Here's how the part is built. I have some questions about the finished solid (model axes, mm). Coordinates: 2 decimals unless noted, no trailing zeros. Write each loop counter-clockwise with the first axis right and the second up, starting at its lowest first coordinate (ties: lowest second). Pieces come first, ordered by that corner, then holes.
Item 1: If we section it at C-C (x = 87.5): Please give me the cut outline in (y, z), then the cut area to 3 significant figures.
Item 2: If we section it at D-D (y = -201): Please give me the cut outline in (x, z), then the cut area to 3 significant figures.
Item 3: If we section it at B-B (z = -5.75): Count the separate pieces of the cut face and the enclosed holes in it, then the cut area to 3 significant figures.
Item 4: If we section it at A-A (y = -51): Please give me the cut outline in (x, z), then the cut area to 3 significant figures.
Item 5: If I drill on line 1 (Y direction, x = -85, z = -8); line 2 (X direction, y = 40, z = -3.5); line 3 (Y direction, x = 7.5, z = -13.5), over which ranges is the centre line in solid material (lowest first)?
Item 6: I'm going to push flat-ended pins straight in: pin 1 Ø3 at (x, z) = (-165, -14) entering from -Y; pin 2 Ø5.5 at (x, z) = (-5.5, -7) entering from +Y; pin 3 Ø5 at (y, z) = (56, -4) entering from -X. Where does each tip first touch, or does it pass through?
from build123d import *

# Parameters (mm, degrees)
F2_DEPTH  = 31.75
F4_DEPTH  = 11.43
F6_DEPTH  = 8.89
F8_DEPTH  = 8.89
F10_DEPTH = 8.89
F12_DEPTH = 8.89
F13_R     = 304.8
F14_DEPTH = 20.32
F16_DEPTH = 10.16
F18_DEPTH = 10.16
F20_DEPTH = 10.16
F22_DEPTH = 10.16
F24_DEPTH = 10.16
F26_DEPTH = 10.16
F27_R     = 304.8
F28_DEPTH = 38.1


with BuildPart() as f2:
    # F1 (on Top) → F2 (new body)
    with BuildSketch(Plane.XY):
        with BuildLine():
            ThreePointArc((-0.430908, 226.982415), (-79.711548, 181.706479), (-169.227302, 163.75488))
            Line((-169.227302, 163.75488), (-169.227302, -60.819823))
            ThreePointArc((-169.227302, -60.819823), (-113.369381, -185.600772), (2.933838, -257.461429))
            ThreePointArc((2.933838, -257.461429), (118.158195, -186.267639), (169.227302, -60.819823))
            Line((169.227302, -60.819823), (169.227302, 166.105464))
            ThreePointArc((169.227302, 166.105464), (79.251051, 182.199338), (-0.430908, 226.982415))
        make_face()
    extrude(amount=F2_DEPTH)

    # F3 (on face) → F4 (cut)
    with BuildSketch(Plane.XY.offset(31.75)):
        with BuildLine():
            ThreePointArc((-0.374756, 195.493162), (-69.015087, 155.212384), (-147.227302, 140.485346))
            Line((-147.227302, 140.485346), (-147.227302, -60.819823))
            ThreePointArc((-147.227302, -60.819823), (-96.87236, -165.644499), (2.548859, -225.97073))
            ThreePointArc((2.548859, -225.97073), (100.066402, -165.452439), (147.227302, -60.819823))
            Line((147.227302, -60.819823), (147.227302, 142.530277))
            ThreePointArc((147.227302, 142.530277), (68.839046, 156.227594), (-0.374756, 195.493162))
        make_face()
        with BuildLine():
            Line((-132.618561, -60.819823), (-135.227293, 127.792969))
            ThreePointArc((-135.227293, 127.792969), (-63.429471, 141.425292), (-0.343994, 178.316891))
            ThreePointArc((-0.343994, 178.316891), (63.444172, 142.853346), (135.227293, 129.670903))
            Line((135.227293, 129.670903), (135.227293, -60.819823))
            ThreePointArc((135.227293, -60.819823), (90.906741, -154.674215), (2.340942, -208.794981))
            ThreePointArc((2.340942, -208.794981), (-88.121088, -155.768197), (-132.618561, -60.819823))
        make_face(mode=Mode.SUBTRACT)
    extrude(amount=-F4_DEPTH, mode=Mode.SUBTRACT)

    # F5 (on face) → F6 (cut)
    with BuildSketch(Plane.XY.offset(31.75)):
        with BuildLine():
            Line((-92.367917, 113.127932), (-45.701414, 36.461424))
            Line((-45.701414, 36.461424), (53.798582, 36.461424))
            Line((53.798582, 36.461424), (100.798585, 113.127932))
            ThreePointArc((100.798585, 113.127932), (80.575922, 103.064845), (63.631594, 88.127926))
            ThreePointArc((63.631594, 88.127926), (53.573391, 92.641146), (42.631593, 91.29443))
            ThreePointArc((42.631593, 91.29443), (54.451081, 69.882064), (36.776334, 52.976649))
            ThreePointArc((36.776334, 52.976649), (17.177594, 68.050279), (25.131593, 91.460936))
            ThreePointArc((25.131593, 91.460936), (17.890886, 96.996315), (8.798584, 97.627439))
            ThreePointArc((8.798584, 97.627439), (11.159805, 118.634697), (4.798584, 138.794437))
            ThreePointArc((4.798584, 138.794437), (-2.905563, 118.768028), (-0.36792, 97.461425))
            ThreePointArc((-0.36792, 97.461425), (-9.949798, 97.0895), (-17.034912, 90.627931))
            ThreePointArc((-17.034912, 90.627931), (-9.141713, 67.277349), (-29.217625, 52.976649))
            ThreePointArc((-29.217625, 52.976649), (-46.671559, 70.152552), (-34.034912, 91.127932))
            ThreePointArc((-34.034912, 91.127932), (-45.151665, 92.60432), (-55.201415, 87.627932))
            ThreePointArc((-55.201415, 87.627932), (-71.812791, 103.251959), (-92.367917, 113.127932))
        make_face()
    extrude(amount=-F6_DEPTH, mode=Mode.SUBTRACT)

    # F7 (on face) → F8 (cut)
    with BuildSketch(Plane.XY.offset(31.75)):
        Polygon((1.882065, 29.461427), (67.46655, -21.70459), (47.798585, 29.461427), align=None)
    extrude(amount=-F8_DEPTH, mode=Mode.SUBTRACT)

    # F9 (on face) → F10 (cut)
    with BuildSketch(Plane.XY.offset(31.75)):
        Polygon((1.048598, 29.461427), (-44.867922, 29.461427), (-64.53491, -21.70459), align=None)
    extrude(amount=-F10_DEPTH, mode=Mode.SUBTRACT)

    # F11 (on face) → F12 (cut)
    with BuildSketch(Plane.XY.offset(31.75)):
        with BuildLine():
            Line((1.246826, -2.287598), (-12.11792, -13.121582))
            Line((-12.11792, -13.121582), (-17.534912, -87.538578))
            Line((-17.534912, -87.538578), (-27.712647, -87.456539))
            ThreePointArc((-27.712647, -87.456539), (-43.153284, -84.398915), (-38.845949, -99.538572))
            Line((-38.845949, -99.538572), (-9.99292, -99.538572))
            Line((-9.99292, -99.538572), (-10.230225, -136.209473))
            Line((-10.230225, -136.209473), (-16.215088, -143.374518))
            Line((-16.215088, -143.374518), (-10.201416, -149.538577))
            Line((-10.201416, -149.538577), (-3.201416, -149.538577))
            ThreePointArc((-3.201416, -149.538577), (-5.538014, -164.476042), (1.798584, -177.695796))
            ThreePointArc((1.798584, -177.695796), (7.646569, -164.237988), (6.611084, -149.601072))
            Line((6.611084, -149.601072), (11.986084, -149.476081))
            Line((11.986084, -149.476081), (19.017333, -143.569827))
            Line((19.017333, -143.569827), (12.298584, -136.203617))
            Line((12.298584, -136.203617), (12.131592, -99.538572))
            Line((12.131592, -99.538572), (41.065186, -99.538572))
            ThreePointArc((41.065186, -99.538572), (45.517328, -84.304241), (29.96753, -87.48389))
            Line((29.96753, -87.48389), (19.965576, -87.538578))
            Line((19.965576, -87.538578), (14.132569, -12.705078))
            Line((14.132569, -12.705078), (1.246826, -2.287598))
        make_face()
    extrude(amount=-F12_DEPTH, mode=Mode.SUBTRACT)

    # F13 (on face) → F14 (join)
    with BuildSketch(Plane.XY):
        with Locations((1.490798, -15.673031)):
            Circle(F13_R)
    extrude(amount=-F14_DEPTH)

    # F15 (on face) → F16 (cut)
    with BuildSketch(Plane.XY):
        with BuildLine():
            Line((-189.547302, 184.049582), (-189.547302, -62.041552))
            ThreePointArc((-189.547302, -62.041552), (-127.393416, -200.419297), (2.747771, -278.360156))
            ThreePointArc((2.747771, -278.360156), (132.255423, -201.050673), (189.547302, -61.527812))
            Line((189.547302, -61.527812), (189.547302, 187.032623))
            ThreePointArc((189.547302, 187.032623), (87.662532, 200.775305), (-0.410603, 253.808226))
            ThreePointArc((-0.410603, 253.808226), (-88.09635, 200.268094), (-189.547302, 184.049582))
        make_face()
        with BuildLine():
            Line((-169.227302, -60.819823), (-169.227302, 163.75488))
            ThreePointArc((-169.227302, 163.75488), (-79.711548, 181.706479), (-0.430908, 226.982415))
            ThreePointArc((-0.430908, 226.982415), (79.251051, 182.199338), (169.227302, 166.105464))
            Line((169.227302, 166.105464), (169.227302, -60.819823))
            ThreePointArc((169.227302, -60.819823), (118.158195, -186.267639), (2.933838, -257.461429))
            ThreePointArc((2.933838, -257.461429), (-113.369381, -185.600772), (-169.227302, -60.819823))
        make_face(mode=Mode.SUBTRACT)
    extrude(amount=-F16_DEPTH, mode=Mode.SUBTRACT)

    # F17 (on face) → F18 (cut)
    with BuildSketch(Plane.XY):
        with BuildLine():
            ThreePointArc((-0.374756, 195.493162), (-69.015087, 155.212384), (-147.227302, 140.485346))
            Line((-147.227302, 140.485346), (-147.227302, -60.819823))
            ThreePointArc((-147.227302, -60.819823), (-96.87236, -165.644499), (2.548859, -225.97073))
            ThreePointArc((2.548859, -225.97073), (100.066402, -165.452439), (147.227302, -60.819823))
            Line((147.227302, -60.819823), (147.227302, 142.530277))
            ThreePointArc((147.227302, 142.530277), (68.839046, 156.227594), (-0.374756, 195.493162))
        make_face()
        with BuildLine():
            Line((-132.618561, -60.819823), (-135.227293, 127.792969))
            ThreePointArc((-135.227293, 127.792969), (-63.429471, 141.425292), (-0.343994, 178.316891))
            ThreePointArc((-0.343994, 178.316891), (63.444172, 142.853346), (135.227293, 129.670903))
            Line((135.227293, 129.670903), (135.227293, -60.819823))
            ThreePointArc((135.227293, -60.819823), (90.906741, -154.674215), (2.340942, -208.794981))
            ThreePointArc((2.340942, -208.794981), (-88.121088, -155.768197), (-132.618561, -60.819823))
        make_face(mode=Mode.SUBTRACT)
    extrude(amount=-F18_DEPTH, mode=Mode.SUBTRACT)

    # F19 (on face) → F20 (cut)
    with BuildSketch(Plane.XY):
        with BuildLine():
            Line((19.965576, -87.538578), (14.132569, -12.705078))
            Line((14.132569, -12.705078), (1.246826, -2.287598))
            Line((1.246826, -2.287598), (-12.11792, -13.121582))
            Line((-12.11792, -13.121582), (-17.534912, -87.538578))
            Line((-17.534912, -87.538578), (-27.712647, -87.456539))
            ThreePointArc((-27.712647, -87.456539), (-43.153284, -84.398915), (-38.845949, -99.538572))
            Line((-38.845949, -99.538572), (-9.99292, -99.538572))
            Line((-9.99292, -99.538572), (-10.230225, -136.209473))
            Line((-10.230225, -136.209473), (-16.215088, -143.374518))
            Line((-16.215088, -143.374518), (-10.201416, -149.538577))
            Line((-10.201416, -149.538577), (-3.201416, -149.538577))
            ThreePointArc((-3.201416, -149.538577), (-5.538014, -164.476042), (1.798584, -177.695796))
            ThreePointArc((1.798584, -177.695796), (7.646569, -164.237988), (6.611084, -149.601072))
            Line((6.611084, -149.601072), (11.986084, -149.476081))
            Line((11.986084, -149.476081), (19.017333, -143.569827))
            Line((19.017333, -143.569827), (12.298584, -136.203617))
            Line((12.298584, -136.203617), (12.131592, -99.538572))
            Line((12.131592, -99.538572), (41.065186, -99.538572))
            ThreePointArc((41.065186, -99.538572), (45.517328, -84.304241), (29.96753, -87.48389))
            Line((29.96753, -87.48389), (19.965576, -87.538578))
        make_face()
    extrude(amount=-F20_DEPTH, mode=Mode.SUBTRACT)

    # F21 (on face) → F22 (cut)
    with BuildSketch(Plane.XY):
        Polygon((1.048598, 29.461427), (-44.867922, 29.461427), (-64.53491, -21.70459), align=None)
    extrude(amount=-F22_DEPTH, mode=Mode.SUBTRACT)

    # F23 (on face) → F24 (cut)
    with BuildSketch(Plane.XY):
        Polygon((47.798585, 29.461427), (1.465576, 29.461427), (67.46655, -21.70459), align=None)
    extrude(amount=-F24_DEPTH, mode=Mode.SUBTRACT)

    # F25 (on face) → F26 (cut)
    with BuildSketch(Plane.XY):
        with BuildLine():
            ThreePointArc((-34.034912, 91.127932), (-45.151665, 92.60432), (-55.201415, 87.627932))
            ThreePointArc((-55.201415, 87.627932), (-71.812791, 103.251959), (-92.367917, 113.127932))
            Line((-92.367917, 113.127932), (-45.701414, 36.461424))
            Line((-45.701414, 36.461424), (53.798582, 36.461424))
            Line((53.798582, 36.461424), (100.798585, 113.127932))
            ThreePointArc((100.798585, 113.127932), (80.575922, 103.064845), (63.631594, 88.127926))
            ThreePointArc((63.631594, 88.127926), (53.573391, 92.641146), (42.631593, 91.29443))
            ThreePointArc((42.631593, 91.29443), (54.451081, 69.882064), (36.776334, 52.976649))
            ThreePointArc((36.776334, 52.976649), (17.177594, 68.050279), (25.131593, 91.460936))
            ThreePointArc((25.131593, 91.460936), (17.890886, 96.996315), (8.798584, 97.627439))
            ThreePointArc((8.798584, 97.627439), (11.159805, 118.634697), (4.798584, 138.794437))
            ThreePointArc((4.798584, 138.794437), (-2.905563, 118.768028), (-0.36792, 97.461425))
            ThreePointArc((-0.36792, 97.461425), (-9.949798, 97.0895), (-17.034912, 90.627931))
            ThreePointArc((-17.034912, 90.627931), (-9.141713, 67.277349), (-29.217625, 52.976649))
            ThreePointArc((-29.217625, 52.976649), (-46.671559, 70.152552), (-34.034912, 91.127932))
        make_face()
    extrude(amount=-F26_DEPTH, mode=Mode.SUBTRACT)

    # F27 (on face) → F28 (cut)
    with BuildSketch(Plane.XY):
        with Locations((1.490798, -15.673031)):
            Circle(F27_R)
    extrude(amount=F28_DEPTH, mode=Mode.SUBTRACT)


solid = f2.part
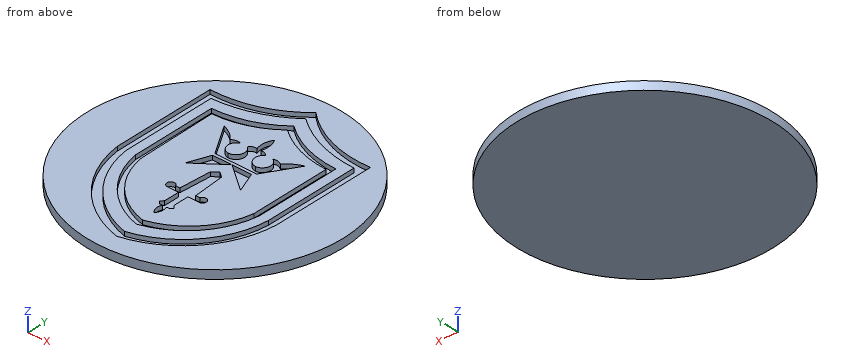
Answer list:
1. outline: (-308.09, -20.32) - (276.74, -20.32) - (276.74, 0) - (200.83, 0) - (200.83, -10.16) - (179.39, -10.16) - (179.39, 0) - (150.4, 0) - (150.4, -10.16) - (135.71, -10.16) - (135.71, 0) - (107.27, 0) - (107.27, -10.16) - (91.44, -10.16) - (91.44, 0) - (-158.36, 0) - (-158.36, -10.16) - (-178.53, -10.16) - (-178.53, 0) - (-216.04, 0) - (-216.04, -10.16) - (-241.36, -10.16) - (-241.36, 0) - (-308.09, 0) - close
1. area: 10,900 mm2
2. outline: (-240.49, -20.32) - (243.48, -20.32) - (243.48, 0) - (132.3, 0) - (132.3, -10.16) - (104.49, -10.16) - (104.49, 0) - (58.94, 0) - (58.94, -10.16) - (25.45, -10.16) - (25.45, 0) - (-22.59, 0) - (-22.59, -10.16) - (-54.83, -10.16) - (-54.83, 0) - (-98.59, 0) - (-98.59, -10.16) - (-126.88, -10.16) - (-126.88, 0) - (-240.49, 0) - close
2. area: 8,600 mm2
3. separate pieces: 3
3. enclosed holes: 6
3. area: 233,000 mm2
4. outline: (-301.26, -20.32) - (304.24, -20.32) - (304.24, 0) - (189.55, 0) - (189.55, -10.16) - (169.23, -10.16) - (169.23, 0) - (147.23, 0) - (147.23, -10.16) - (135.23, -10.16) - (135.23, 0) - (17.12, 0) - (17.12, -10.16) - (-14.88, -10.16) - (-14.88, 0) - (-132.75, 0) - (-132.75, -10.16) - (-147.23, -10.16) - (-147.23, 0) - (-169.23, 0) - (-169.23, -10.16) - (-189.55, -10.16) - (-189.55, 0) - (-301.26, 0) - close
4. area: 11,300 mm2
5. line 1: y = -307.94 to -238.46, -212.94 to -177.69, -159.1 to 101.02, 110.46 to 134.62, 149.88 to 179.78, 201.43 to 276.6
5. line 2: x = -298.18 to -189.55, -169.23 to -147.23, -134.01 to -47.86, 55.97 to 135.23, 147.23 to 169.23, 189.55 to 301.16
5. line 3: y = -320.41 to 289.07
6. pin 1: stops at y = -271.96
6. pin 2: stops at y = 289.1
6. pin 3: stops at x = -295.36
